Read the model definition and answer for the solid it produces. Units are mm, in the model's axes. A direction names the side the tool comes from. Coordinates: 2 decimals unless noted, no trailing zeros. Order: outer loops, then holes, each group sorted by start corner. A loop starts at its lowest first (then second) coordinate and runs counter-clockwise, first axis right, second up.
from build123d import *

# Parameters (mm, degrees)
F1_DEPTH = 127
F2_DEPTH = 50.8
F0_R     = 50.8
F3_DEPTH = 25.4
F4_DEPTH = 50.8


with BuildPart() as f1:
    # F0 (on Front) → F1 (new body)
    with BuildSketch(Plane.XZ):
        Polygon((254, 0), (0, 0), (0, -63.5), (79.8352242538, -63.5), (41.7352242538, -25.4), (211.6168698438, -25.4), (190.5, -63.5), (254, -63.5), align=None)
    extrude(amount=F1_DEPTH)

    # F0 (on Front) → F2 (join)
    with BuildSketch(Plane.XZ):
        with BuildLine():
            Line((40.1998028961, 119.7350906188), (0, 0))
            Line((0, 0), (254, 0))
            Line((254, 0), (207.6520293862, 122.8259365118))
            ThreePointArc((207.6520293862, 122.8259365118), (211.9338340509, 107.391873178), (213.3767146031, 91.44))
            ThreePointArc((213.3767146031, 91.44), (110.1415733543, 3.7033843519), (40.1998028961, 119.7350906188))
        make_face()
    extrude(amount=F2_DEPTH)

    # F0 (on Front) → F3 (join)
    with BuildSketch(Plane.XZ):
        with BuildLine():
            ThreePointArc((207.6520293862, 122.8259365118), (122.8360711229, 180.3248597286), (40.1998028961, 119.7350906188))
            ThreePointArc((40.1998028961, 119.7350906188), (110.1415733543, 3.7033843519), (213.3767146031, 91.44))
            ThreePointArc((213.3767146031, 91.44), (211.9338340509, 107.391873178), (207.6520293862, 122.8259365118))
        make_face()
        with Locations((124.4767146031, 91.44)):
            Circle(F0_R, mode=Mode.SUBTRACT)
    extrude(amount=F3_DEPTH)

    # F4 (add): a face of the model
    f4_faces = [f1.faces().sort_by_distance(p)[0] for p in [
        (122.8824755281, -25.4, 177.8108162462),
    ]]
    extrude(f4_faces, amount=F4_DEPTH)


solid = f1.part
Q1. The part is cut by section C-C, the plane y = -36.5. Determine the outline of the cut face in (x, z).
Q2. Straight lines are drawn through the part: L1, parallel to Z at x = 122.5, y = -58; L2, parallel to Y at x = 32.5, z = 25; L3, parallel to Y at x = 60, z = 79.5. For each, find the intervals that lie inside material, in ascending order.
Q3. Which of the six approach directions +Z, -Z, +X, -X, +Y, -Y give full straight-line access (tool end or side, diameter ignored) to faces 4 (the flat face through (129, -88, 0)), 5 (the flat face through (254, -63, -32)), 6 (the flat face through (125, -63, -25.4)), 7 (the flat face through (117, -50.8, 2.6)), 8 (the flat face through (163, -76.2, 53))?
Q4. Determine the mould class of faces 1 (the flat face through (231.15, -25.04, 60.55)), 2 (the flat face through (201.21, -62.61, -44.18)), 3 (the flat face through (125, 0, 33)) for opening direction Z: +Z half, -Z half, draft (parallel to the pull), parting line (faces both ways), or undercut.
Q5. The part is cut by section D-D, the plane x = 86. Determine the outline of the cut face in (y, z), then the cut area to 3 significant figures.
Q6. The part is cut by section A-A, the plane y = -70. Determine the outline of the cut face in (x, z), then the cut area to 3 significant figures.
Q7. Each of these flat-tipped pins is pushed along its axis until it touches: P1, Ø1.5, axis at x = 96, y = -104.5, coming from the +Z side; P2, Ø8, axis at y = -78.5, z = 143, coming from the +X side; P3, Ø1.5, axis at y = -70, z = 57, coming from the -X side. Where does it stop, or does it pass through?
Q8. The part is cut by section B-B, the plane z = 64. Determine the outline of the cut face in (x, y).
Computed values:
1. outline: (0, -63.5) - (79.84, -63.5) - (41.74, -25.4) - (211.62, -25.4) - (190.5, -63.5) - (254, -63.5) - (254, 0) - (207.65, 122.83) arc R88.9 ccw to (40.2, 119.74) - (0, 0) - close; hole circle Ø101.6 at (124.48, 91.44)
2. L1: z = -25.4 to 0, 2.56 to 40.68, 142.2 to 180.32
2. L2: y = -50.8 to 0
2. L3: y = -76.2 to 0
3. face 4: +X, -X, -Y
3. face 5: +Z, -Z, +X, +Y, -Y
3. face 6: +Y, -Y
3. face 7: -Y
3. face 8: +Z, +X, -X, -Y
4. face 1: +Z half
4. face 2: undercut
4. face 3: draft
5. outline: (-127, -25.4) - (0, -25.4) - (0, 58.27) - (-76.2, 58.27) - (-76.2, 11.3) - (-50.8, 11.3) - (-50.8, 0) - (-127, 0) - close; (-76.2, 124.61) - (0, 124.61) - (0, 171.58) - (-76.2, 171.58) - close
5. area: 11,000 mm2
6. outline: (0, -63.5) - (79.84, -63.5) - (41.74, -25.4) - (211.62, -25.4) - (190.5, -63.5) - (254, -63.5) - (254, 0) - (0, 0) - close; circle Ø177.8 at (124.48, 91.44); hole circle Ø101.6 at (124.48, 91.44)
6. area: 27,500 mm2
7. P1: stops at z = 0
7. P2: stops at x = 199.12
7. P3: stops at x = 42.21
8. outline: (21.49, -50.8) - (39.92, -50.8) - (39.92, -76.2) - (81.73, -76.2) - (81.73, 0) - (21.49, 0) - close; (167.23, -76.2) - (209.04, -76.2) - (209.04, -50.8) - (229.85, -50.8) - (229.85, 0) - (167.23, 0) - close
